```python
from build123d import *

# Parameters (mm, degrees)
CROQUIS2_R              = 0.8
CROQUIS2_R_2            = 3.04
SALIENTE_EXTRUIR1_DEPTH = 1
REDONDEO1_R             = 1


with BuildPart() as part:
    # Croquis2 → Saliente-Extruir1 (new, symmetric)
    with BuildSketch(Plane(origin=(0, 0, 0), x_dir=(1, 0, 0), z_dir=(0, 1, 0))):
        with BuildLine():
            Line((-2.781654184, 3.52), (-5.006977531, -15.824))
            ThreePointArc((-5.006977531, -15.824), (0, -21.44), (5.006977531, -15.824))
            Line((5.006977531, -15.824), (2.781654184, 3.52))
            ThreePointArc((2.781654184, 3.52), (0, 6), (-2.781654184, 3.52))
        make_face()
        with Locations(Location((0, 0, 0), (0, 0, 270))):
            Circle(CROQUIS2_R, mode=Mode.SUBTRACT)
        with Locations(Location((0, 3.2, 0), (0, 0, 270))):
            Circle(CROQUIS2_R, mode=Mode.SUBTRACT)
        with Locations(Location((0, -16.4, 0), (0, 0, 270))):
            Circle(CROQUIS2_R_2, mode=Mode.SUBTRACT)
    extrude(amount=SALIENTE_EXTRUIR1_DEPTH, both=True)

    # Redondeo1
    redondeo1_edges = [part.edges().sort_by_distance(p)[0] for p in [
        (-3.894315858, -1, 6.152),
        (0, -1, -6),
        (3.894315858, -1, 6.152),
        (-3.894315858, 1, 6.152),
        (0, 1, -6),
        (3.894315858, 1, 6.152),
        (0, -1, 21.44),
        (0, 1, 21.44),
    ]]
    fillet(redondeo1_edges, radius=REDONDEO1_R - 0.0001)  # a hair under: the kernel refuses the full size


solid = part.part
```
The listing builds one solid part. Answer for the finished solid, in the listing's coordinates (mm). Give positions to 0.01 mm unless a question says otherwise; leave off trailing zeros.
Item 1: For a pull along Z with two mould halves and no side action, classify faces 1 (the face through (0, 1, 8)), 2 (the face through (3.595, 0.699, 6.049)), 3 (the face through (0, 0, -4)) as pulls with the +Z half, pulls with the -Z half, needs draft (parallel to the pull), parting line crosses it, or undercut.
From the geometry:
face 1: needs draft
face 2: pulls with the -Z half
face 3: undercut
Item 2: Find the intervals of material crossed by probe 1 along Z at (x, y) = (-0.25, -0.45); probe 2 along X at (y, z) = (-0.1, 16.4) (3 decimals); probe 3 along Z at (x, y) = (-0.5, 0.1), in increasing order.
From the geometry:
probe 1: z = -5.88 to -3.96, -2.44 to -0.76, 0.76 to 13.37, 19.43 to 21.33
probe 2: x = -5.035 to -3.04, 3.04 to 5.035
probe 3: z = -5.95 to -3.82, -2.58 to -0.62, 0.62 to 13.4, 19.4 to 21.41
Item 3: The part is cut by section A-A, the plane x = 0. Count the separate pieces of the cut face and the enclosed holes in it, and give its area (3 significant figures).
From the geometry:
separate pieces: 4
enclosed holes: 0
area: 35.5 mm2
